Model file for the job. Use its own axes, mm. Face numbers are marked on the shaded views. A direction names the side the tool comes from. Give positions to 0.01 mm unless a question says otherwise; leave off trailing zeros. Write each loop counter-clockwise with the first axis right and the second up, starting at its lowest first coordinate (ties: lowest second). Pieces come first, ordered by that corner, then holes. Notation, with made-up numbers: (2.25, 4.25) - (18.25, 4.25) arc R26 cw to (18.25, 40.25) - close; hole circle Ø2 at (-16.5, 20.25). An arc over 180 degrees is marked (long way). One line per item, written item: value. Start each with the question number.
(1) Cut at B-B, the plane y = -27. List the corners of the cut face in (x, z), and give its area (3 significant figures).
(2) Drop flat-ended pins along their axis: P1, Ø4, axis at x = -21.5, z = -15, coming from the -Y side; P2, Ø10.5, axis at x = -20, z = -13.5, coming from the -Y side; P3, Ø5.5, axis at x = -15, y = -36, coming from the -Z side. Give the stop position or say it passes through.
(3) Cut at D-D, the plane y = -23. List the corners of the cut face in (x, z).
(4) Probe L1, parallel to Y at x = -30, z = -9.25; L2, parallel to Y at x = -20.75, z = -9.25; L3, parallel to Y at x = -16.5, z = -4.5. List the from-to ranges inside material, lowest first.
(5) 3-axis set-ups, long thin cutter, end or side, ignore diameter. For the marked faces 1, 2, 3 and 4: which of +Z, -Z, +X, -X, +Y, -Y reach the whole face in a straight line?
(6) Cut at C-C, the plane x = -30. List the corners of the cut face in (y, z), and give its area (3 significant figures).
(7) Cut at A-A, the plane z = -2.5. List the corners of the cut face in (x, y), and give its area (3 significant figures).
(8) Mould opens along Y. For the marked faces 5, 6 and 7 say: pulls with the +Y half, pulls with the -Y half, needs draft (parallel to the pull), parting line crosses it, or undercut.
from build123d import *

# Parameters (mm, degrees)
CYLINDER040_R          = 1.75
CYLINDER040_DEPTH      = 44
CYLINDER040_ROLL_ANGLE = 90
CYLINDER049_R          = 2
CYLINDER049_DEPTH      = 42
CYLINDER051_R          = 1.5
CYLINDER051_DEPTH      = 42
CYLINDER053_R          = 4
CYLINDER053_DEPTH      = 4
CYLINDER053_ROLL_ANGLE = 90
CYLINDER054_R          = 4
CYLINDER054_DEPTH      = 4
CYLINDER054_ROLL_ANGLE = 90
BOX089_W               = 42
BOX089_H               = 3
BOX089_DEPTH           = 3
CYLINDER043_R          = 1.75
CYLINDER043_DEPTH      = 44
CYLINDER043_ROLL_ANGLE = 90
CYLINDER048_R          = 3.4
CYLINDER048_DEPTH      = 25
BOX084_W               = 3
BOX084_H               = 14.6
BOX084_DEPTH           = 25
BOX085_W               = 7
BOX085_H               = 10.6
BOX085_DEPTH           = 3.5
CHAMFER_SIZE           = 4
BOX080_W               = 15
BOX080_H               = 4.6
BOX080_DEPTH           = 25


with BuildPart() as cylinder_for_hole_3_motherboard003:
    # Cylinder040 → Cylinder040 (new body)
    with BuildSketch(Plane.XY):
        Circle(CYLINDER040_R)
    extrude(amount=CYLINDER040_DEPTH)


with BuildPart() as cylinder_for_hole_3_motherboard003_1:
    # Cylinder040 roll: moved
    add(cylinder_for_hole_3_motherboard003.part.rotate(Axis((0, 0, 0), (1, 0, 0)), CYLINDER040_ROLL_ANGLE))


with BuildPart() as cylinder_for_hole_3_motherboard003_2:
    # Cylinder040 placement: moved
    add(cylinder_for_hole_3_motherboard003_1.part.moved(Location((-20, 6, -13.5))))


with BuildPart() as blower_screw:
    # Cylinder049 → Cylinder049 (new body)
    with BuildSketch(Plane(origin=(-30, -23, -19), x_dir=(1, 0, 0), z_dir=(0, 0, 1))):
        Circle(CYLINDER049_R)
    extrude(amount=CYLINDER049_DEPTH)


with BuildPart() as extruder_screw_l:
    # Cylinder051 → Cylinder051 (new body)
    with BuildSketch(Plane(origin=(-14.2, -35.8, -8), x_dir=(1, 0, 0), z_dir=(0, 0, 1))):
        Circle(CYLINDER051_R)
    extrude(amount=CYLINDER051_DEPTH)


with BuildPart() as cylinder053:
    # Cylinder053 → Cylinder053 (new body)
    with BuildSketch(Plane.XY):
        Circle(CYLINDER053_R)
    extrude(amount=CYLINDER053_DEPTH)


with BuildPart() as cylinder053_1:
    # Cylinder053 roll: moved
    add(cylinder053.part.rotate(Axis((0, 0, 0), (1, 0, 0)), CYLINDER053_ROLL_ANGLE))


with BuildPart() as cylinder053_2:
    # Cylinder053 placement: moved
    add(cylinder053_1.part.moved(Location((-20, -20, -2.5))))


with BuildPart() as cylinder054:
    # Cylinder054 → Cylinder054 (new body)
    with BuildSketch(Plane.XY):
        Circle(CYLINDER054_R)
    extrude(amount=CYLINDER054_DEPTH)


with BuildPart() as cylinder054_1:
    # Cylinder054 roll: moved
    add(cylinder054.part.rotate(Axis((0, 0, 0), (1, 0, 0)), CYLINDER054_ROLL_ANGLE))


with BuildPart() as cylinder054_2:
    # Cylinder054 placement: moved
    add(cylinder054_1.part.moved(Location((-20, -20, -13.5))))


with BuildPart() as fastener_hole001:
    # Box089 → Box089 (new body)
    with BuildSketch(Plane(origin=(-21.5, -28.2, -17.5), x_dir=(1, 0, 0), z_dir=(0, 0, 1))):
        with Locations((21, 1.5)):
            Rectangle(BOX089_W, BOX089_H)
    extrude(amount=BOX089_DEPTH)


with BuildPart() as blower_retention_holes:
    # Cylinder043 → Cylinder043 (new body)
    with BuildSketch(Plane.XY):
        Circle(CYLINDER043_R)
    extrude(amount=CYLINDER043_DEPTH)


with BuildPart() as blower_retention_holes_1:
    # Cylinder043 roll: moved
    add(blower_retention_holes.part.rotate(Axis((0, 0, 0), (1, 0, 0)), CYLINDER043_ROLL_ANGLE))


with BuildPart() as blower_retention_holes_2:
    # Cylinder043 placement: moved
    add(blower_retention_holes_1.part.moved(Location((-20, 6, -2.5))))

    # Fusion023: union cylinder for hole 3 - Motherboard003, blower screw, extruder screw  L, Cylinder053, Cylinder054, fastener hole001
    add(cylinder_for_hole_3_motherboard003_2.part)
    add(blower_screw.part)
    add(extruder_screw_l.part)
    add(cylinder053_2.part)
    add(cylinder054_2.part)
    add(fastener_hole001.part)


with BuildPart() as blower_retention:
    # Cylinder048 → Cylinder048 (new body)
    with BuildSketch(Plane(origin=(-30, -23, -19), x_dir=(1, 0, 0), z_dir=(0, 0, 1))):
        Circle(CYLINDER048_R)
    extrude(amount=CYLINDER048_DEPTH)


with BuildPart() as motor_bracket_base_l_lower:
    # Box084 → Box084 (new body)
    with BuildSketch(Plane(origin=(-17.5, -30.2, -19), x_dir=(1, 0, 0), z_dir=(0, 0, 1))):
        with Locations((1.5, 7.3)):
            Rectangle(BOX084_W, BOX084_H)
    extrude(amount=BOX084_DEPTH)


with BuildPart() as motor_bracket_base_l_upper_chamfered:
    # Box085 → Box085 (new body)
    with BuildSketch(Plane(origin=(-17.5, -40.2, 2.5), x_dir=(1, 0, 0), z_dir=(0, 0, 1))):
        with Locations((3.5, 5.3)):
            Rectangle(BOX085_W, BOX085_H)
    extrude(amount=BOX085_DEPTH)

    # Chamfer
    chamfer_edges = [motor_bracket_base_l_upper_chamfered.edges().sort_by_distance(p)[0] for p in [
        (-10.5, -29.6, 4.25),
    ]]
    chamfer(chamfer_edges, length=CHAMFER_SIZE)


with BuildPart() as blower_retention_arm_with_holes:
    # Box080 → Box080 (new body)
    with BuildSketch(Plane(origin=(-32.5, -20.2, -19), x_dir=(1, 0, 0), z_dir=(0, 0, 1))):
        with Locations((7.5, 2.3)):
            Rectangle(BOX080_W, BOX080_H)
    extrude(amount=BOX080_DEPTH)

    # Fusion022: union blower retention, motor bracket base L lower, motor bracket base L upper chamfered
    add(blower_retention.part)
    add(motor_bracket_base_l_lower.part)
    add(motor_bracket_base_l_upper_chamfered.part)

    # Cut013: cut blower retention holes
    add(blower_retention_holes_2.part, mode=Mode.SUBTRACT)


solid = blower_retention_arm_with_holes.part
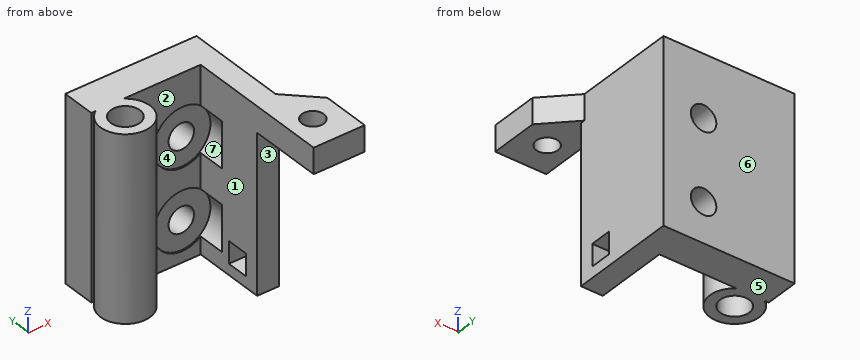
Answers follow:
1. outline: (-17.5, -19) - (-14.5, -19) - (-14.5, -17.5) - (-17.5, -17.5) - close; (-17.5, -14.5) - (-14.5, -14.5) - (-14.5, 6) - (-17.5, 6) - close
1. area: 66.0 mm²
2. P1: stops at y = -20.2
2. P2: stops at y = -30.2
2. P3: stops at z = 2.5
3. outline: (-33.4, -19) - (-32, -19) - (-32, 6) - (-33.4, 6) - close; (-28, -19) - (-26.6, -19) - (-26.6, 6) - (-28, 6) - close; (-17.5, -19) - (-14.5, -19) - (-14.5, 6) - (-17.5, 6) - (-17.5, 0.62) arc R4 cw to (-17.5, -5.62) - (-17.5, -10.38) arc R4 cw to (-17.5, -16.62) - close
4. L1: y = -26.4 to -25, -21 to -15.6
4. L2: y = -20.2 to -15.6
4. L3: y = -30.2 to -15.6
5. face 1: +Z, -Z, -Y
5. face 2: +Z, -Z
5. face 3: -Z, +X, -X, -Y
5. face 4: none
6. outline: (-26.4, -19) - (-25, -19) - (-25, 6) - (-26.4, 6) - close; (-21, -19) - (-15.6, -19) - (-15.6, 6) - (-21, 6) - close
6. area: 170 mm²
7. outline: (-32.5, -20.2) - (-31.93, -20.2) arc R3.4 ccw (long way) to (-28.07, -20.2) - (-24, -20.2) - (-24, -20) - (-21.75, -20) - (-21.75, -15.6) - (-32.5, -15.6) - close; (-18.25, -20) - (-16, -20) - (-16, -24) - (-17.5, -24) - (-17.5, -30.2) - (-14.5, -30.2) - (-14.5, -15.6) - (-18.25, -15.6) - close; hole circle Ø4 at (-30, -23)
7. area: 112 mm²
8. face 5: needs draft
8. face 6: pulls with the +Y half
8. face 7: undercut
